```python
from build123d import *

# Parameters (mm, degrees)
F0_W     = 50.8
F0_H     = 12.7
F0_W_2   = 38.1
F0_H_2   = 7.62
F1_DEPTH = 2.54
F2_DEPTH = 63.5
F4_DEPTH = 50.8
F5_R     = 1.26999
F6_R     = 3.175
F7_DEPTH = 12.7
F8_SIZE  = 0.635


# Not quite as in the source:
# - a fillet or chamfer is up to 0.001 mm smaller than in the source, because OpenCascade refuses the exact size


with BuildPart() as f1:
    # F0 (on Top) → F1 (new body)
    with BuildSketch(Plane.XY):
        Rectangle(F0_W, F0_H)
        Rectangle(F0_W_2, F0_H_2, mode=Mode.SUBTRACT)
        Rectangle(F0_W_2, F0_H_2)
    extrude(amount=-F1_DEPTH)

    # F0 (on Top) → F2 (join)
    with BuildSketch(Plane.XY):
        Rectangle(F0_W, F0_H)
        Rectangle(F0_W_2, F0_H_2, mode=Mode.SUBTRACT)
    extrude(amount=F2_DEPTH)

    # F3 (on Right) → F4 (cut, symmetric)
    with BuildSketch(Plane.YZ):
        Polygon((-17.6573935896, 70.3983381391), (-13.9353135601, 40.1254184544), (17.3301566392, 70.3983381391), align=None)
    extrude(amount=F4_DEPTH, both=True, mode=Mode.SUBTRACT)

    # F5 (radius 1.27 in the source; OpenCascade refuses exactly that, so slightly less here)
    f5_edges = [f1.edges().sort_by_distance(p)[0] for p in [
        (25.4, -6.35, 22.464965),
        (0, -6.35, -2.54),
        (25.4, 0, -2.54),
        (-25.4, 0, -2.54),
        (-25.4, -6.35, 22.464965),
        (0, -6.35, 47.469929),
        (0, -3.81, 49.929295),
        (19.05, 0, 53.618343),
        (0, 3.81, 57.307391),
        (-19.05, 0, 53.618343),
        (-25.4, 0, 53.618343),
        (25.4, 0, 53.618343),
    ]]
    fillet(f5_edges, radius=F5_R)

    # F6 (on Front) → F7 (cut, symmetric)
    with BuildSketch(Plane.XZ):
        with Locations((-10.16, 52.6016924392)):
            Circle(F6_R)
        with Locations((10.16, 52.6016924392)):
            Circle(F6_R)
    extrude(amount=F7_DEPTH, both=True, mode=Mode.SUBTRACT)

    # F8
    f8_edges = [f1.edges().sort_by_distance(p)[0] for p in [
        (-13.335, 3.81, 52.601692),
        (6.985, 3.81, 52.601692),
    ]]
    chamfer(f8_edges, length=F8_SIZE)


solid = f1.part
```
The listing builds one solid part. Answer for the finished solid, in the listing's coordinates (mm). A direction names the side the tool comes from. Coordinates: 2 decimals unless noted, no trailing zeros. Write each loop counter-clockwise with the first axis right and the second up, starting at its lowest first coordinate (ties: lowest second). Pieces come first, ordered by that corner, then holes. Notation, with made-up numbers: (5, 41.25) - (36, 41.25) arc R7 cw to (36, 49.25) - close; hole circle Ø1 at (37.25, -6.5). An arc over 180 degrees is marked (long way). One line per item, written item: value.
1) For a pull along Y with two mould halves and no side action, classify faces 1 (the flat face through (-19.05, 0, 27)), 2 (the cylindrical face through (25.02, 0.36, 53.46)), 3 (the flat face through (0, 3.81, 28)), 4 (the flat face through (0, 1, -2.54)) as pulls with the +Y half, pulls with the -Y half, needs draft (parallel to the pull), parting line crosses it, or undercut.
Geometry check:
face 1: undercut
face 2: pulls with the -Y half
face 3: undercut
face 4: needs draft
2) Find section B-B (z = 25.5). Give the vertices of the cut face in (x, y).
Geometry check:
outline: (-25.4, -5.08) arc R1.27 ccw to (-24.13, -6.35) - (24.13, -6.35) arc R1.27 ccw to (25.4, -5.08) - (25.4, 6.35) - (-25.4, 6.35) - close; hole (-19.05, -3.81) - (19.05, -3.81) - (19.05, 3.81) - (-19.05, 3.81) - close
3) Consider line 1 along Y through (x, z) = (-14.5, 33.5); line 2 along X through (y, z) = (0.25, 47); line 3 along X through (y, z) = (4, 54.5). Determine where each line is inside the solid, lowest interval first. Write a range as from..to.
Geometry check:
line 1: y = -6.35..-3.81, 3.81..6.35
line 2: x = -25.4..-19.05, 19.05..25.4
line 3: x = -25.4..-13.24, -7.08..7.08, 13.24..25.4
4) Each of these flat-tipped pins is pushed along its axis until it touches: pin 1 Ø5 at (x, z) = (-10.16, 52.6) entering from +Y; pin 2 Ø2 at (x, z) = (-17.5, 49) entering from -Y. Where does it stop, or does it pass through?
Geometry check:
pin 1: passes through
pin 2: stops at y = -5.77
5) A tool of negligible diameter and unlimited length cuts with its end or side. For faces 5 (the cylindrical face through (9.75, 5.38, 55.75)), 6 (the flat face through (0, 0, 0)), from which of +Z, -Z, +X, -X, +Y, -Y can it reach the whole face along a straight path? Write none if from no direction.
Geometry check:
face 5: +Y, -Y
face 6: +Z
